Input: part model. Units: mm. Frame: model coordinates. Give positions to 0.01 mm unless a question says otherwise; leave off trailing zeros. Order: outer loops, then holes, each group sorted by start corner. A loop starts at its lowest first (then second) coordinate and runs counter-clockwise, first axis right, second up. Notation, with made-up numbers: (78, 57) - (122, 57) arc R20 ccw to (122, 89) - close; hole circle Ø10 at (-32.75, -12). An arc over 180 degrees is marked (long way). Answer in a Markdown table with one row per item. Add a question column.
1. Ray query, line 1 (X direction, y = -57, z = 1.25); line 2 (Y direction, x = 54.5, z = 1.75); line 3 (Y direction, x = 66.5, z = 1.75). Return the intervals inside material, ascending. Write a range as [from, to].
2. Contact query for flat-ended pins moving along their axis: pin 1 (6 mm diameter, centred on y = -19.5, z = -3.5, fed in from -X); pin 2 (8 mm diameter, centred on x = -33, z = 0.5, fed in from -Y); pin 3 (4 mm diameter, centred on x = -56.57, y = -56.57, fed in from +Z); pin 4 (1.5 mm diameter, centred on y = 35, z = 1, fed in from +X). Output: stop coordinate, or through.
3. Section query A-A on y = -25.5. Return loops of the section in (x, z).
4. Section query B-B on z = -3.75. Return loops of the section in (x, y).
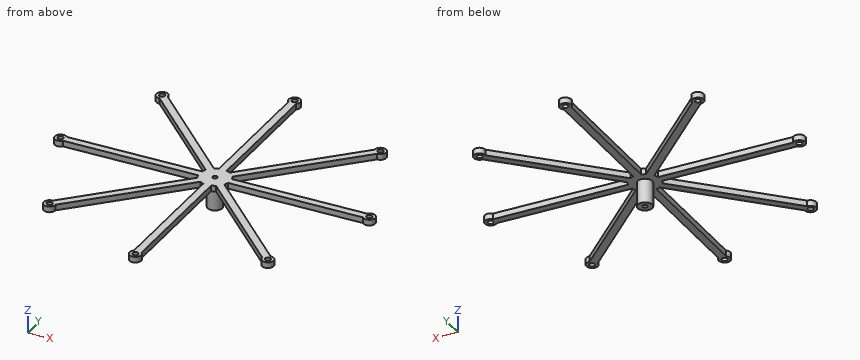
```python
from build123d import *

# Parameters (mm, degrees)
SKETCH_1_R               = 8
EXTRUDE_1_DEPTH          = 3
SKETCH_2_R               = 1.5
EXTRUDE_760_DEPTH        = 3
PATTERN_CIRCULAR_3_COUNT = 8
SKETCH_3_R               = 3.8
EXTRUDE_3_DEPTH          = 12.5
SKETCH_4_R               = 1.25
CUT_EXTRUDE_1_DEPTH      = 119.398690871


with BuildPart() as part:
    # 草图1 → 凸台-拉伸1 (new body)
    with BuildSketch(Plane.XY):
        Circle(SKETCH_1_R)
    extrude(amount=EXTRUDE_1_DEPTH)

    # 草图2 → Extrude 760 (add)
    with BuildSketch(Plane.XY.offset(3)):
        with BuildLine():
            ThreePointArc((7.745966692, 2), (8, 0), (7.745966692, -2))
            Line((7.745966692, -2), (77.763932023, -2))
            ThreePointArc((77.763932023, -2), (83, 0), (77.763932023, 2))
            Line((77.763932023, 2), (7.745966692, 2))
        make_face()
        with Locations((80, 0)):
            Circle(SKETCH_2_R, mode=Mode.SUBTRACT)
    extrude_760 = extrude(amount=-EXTRUDE_760_DEPTH)

    # 阵列(圆周)3: Extrude 760 ×8 about axis
    pattern_circular_3_axis = Axis((0, 0, 0), (0, 0, 1))
    for i in range(1, PATTERN_CIRCULAR_3_COUNT):
        add(extrude_760.rotate(pattern_circular_3_axis, i * 360 / PATTERN_CIRCULAR_3_COUNT))

    # 草图3 → 凸台-拉伸3 (add)
    with BuildSketch(Plane(origin=(0, 0, 0), x_dir=(-1, 0, 0), z_dir=(0, 0, -1))):
        with Locations(Location((0, 0, 0), (0, 0, 180))):
            Circle(SKETCH_3_R)
    extrude(amount=EXTRUDE_3_DEPTH)

    # 草图4 → 切除-拉伸1 (cut, through all)
    with BuildSketch(Plane(origin=(0, 0, -12.5), x_dir=(-1, 0, 0), z_dir=(0, 0, -1))):
        Circle(SKETCH_4_R)
    extrude(amount=-CUT_EXTRUDE_1_DEPTH, mode=Mode.SUBTRACT)


solid = part.part
```
Answer:
| question | item | result |
|---|---|---|
| 1 | line 1 | x = [-59.54, -58.01], [-55.13, -53.6], [-2, 2], [53.6, 55.13], [58.01, 59.54] |
| 1 | line 2 | y = [-58.74, -51.67], [-2, 2], [51.67, 58.74] |
| 1 | line 3 | y = [-2, 2] |
| 2 | pin 1 | passes through |
| 2 | pin 2 | stops at y = -39.83 |
| 2 | pin 3 | stops at z = 3 |
| 2 | pin 4 | stops at x = 38.58 |
| 3 | outline | (-28.33, 0) - (-22.67, 0) - (-22.67, 3) - (-28.33, 3) - close; (-2, 0) - (2, 0) - (2, 3) - (-2, 3) - close; (22.67, 0) - (28.33, 0) - (28.33, 3) - (22.67, 3) - close |
| 4 | outline | circle Ø7.6 at (0, 0); hole circle Ø2.5 at (0, 0) |
